```python
from build123d import *

# Parameters (mm, degrees)
BEAM_SCALE_X           = 1
BEAM_SCALE_Y           = 4
BEAM_SCALE_Z           = 1
LENGTH_SCALE_X         = 10
LENGTH_SCALE_Y         = 1
LENGTH_SCALE_Z         = 1
SKETCH6_W              = 123.825
SKETCH6_H              = 68.58
PAYLOAD_BAY_DEPTH      = 51.8000001
PAYLOAD_BAY_DEPTH_BACK = 63.5
SKETCH16_R             = 5.08
MAST_HOLE_DEPTH        = 51.8000001
MAST_HOLE_DEPTH_BACK   = 101.6
SKETCH15_2_W           = 508
SKETCH15_2_H           = 203.2
LAYER_2_DEPTH          = 50.8


with BuildPart() as part:
    # YZ Section_depthOnly → Depth (revolve)
    with BuildSketch(Plane(origin=(0, 0, 0), x_dir=(0, 0, -1), z_dir=(1, 0, 0))):
        with BuildLine():
            Line((0, 0), (0, -25.4))
            add(Edge.make_bspline(
                [(0, -25.4), (101.6, -14.816666667), (101.6, 0)],
                knots=[5.507991934, 5.507991934, 5.507991934, 6.283185307, 6.283185307, 6.283185307], degree=2, weights=[1, 0.9258201, 1]))
            Line((101.6, 0), (0, 0))
        make_face()
    revolve(axis=Axis((0, 0, 254), (0, 0, -1)))

    # Sketch13 → Height (revolve)
    with BuildSketch(Plane(origin=(0, 0, 0), x_dir=(0, 0, -1), z_dir=(1, 0, 0))):
        with BuildLine():
            Line((0, 0), (-50.8, 0))
            add(Edge.make_bspline(
                [(-50.8, 0), (-50.8, -23.988888889), (0, -25.4)],
                knots=[0, 0, 0, 1.511938821, 1.511938821, 1.511938821], degree=2, weights=[1, 0.727606875, 1]))
            Line((0, -25.4), (0, 0))
        make_face()
    revolve(axis=Axis((0, 0, 0), (0, 0, 1)))


with BuildPart() as part_1:
    # Beam: scaled about (0, 0, 0)
    add(part.part.scale((BEAM_SCALE_X, BEAM_SCALE_Y, BEAM_SCALE_Z), about=(0, 0, 0)))


with BuildPart() as part_2:
    # Length: scaled about (0, 0, 0)
    add(part_1.part.scale((LENGTH_SCALE_X, LENGTH_SCALE_Y, LENGTH_SCALE_Z), about=(0, 0, 0)))

    # Sketch6 → Payload Bay (cut, two sides)
    with BuildSketch(Plane.XY) as payload_bay_sk:
        with Locations((-74.6125, 0)):
            Rectangle(SKETCH6_W, SKETCH6_H)
        with Locations((74.6125, 0)):
            Rectangle(SKETCH6_W, SKETCH6_H)
    extrude(amount=PAYLOAD_BAY_DEPTH, mode=Mode.SUBTRACT)
    extrude(payload_bay_sk.sketch, amount=-PAYLOAD_BAY_DEPTH_BACK, mode=Mode.SUBTRACT)

    # Sketch16 → Mast Hole (cut, two sides)
    with BuildSketch(Plane.XY) as mast_hole_sk:
        Circle(SKETCH16_R)
    extrude(amount=MAST_HOLE_DEPTH, mode=Mode.SUBTRACT)
    extrude(mast_hole_sk.sketch, amount=-MAST_HOLE_DEPTH_BACK, mode=Mode.SUBTRACT)


with BuildPart() as body_2:
    # Sketch15_2 → Layer 2 (new body)
    with BuildSketch(Plane.XY):
        Rectangle(SKETCH15_2_W, SKETCH15_2_H)
    extrude(amount=-LAYER_2_DEPTH)


with BuildPart() as part_3:
    add(part_2.part)

    # Layer 2 Body: intersect body 2
    add(body_2.part, mode=Mode.INTERSECT)


solid = part_3.part
```
Build history of the part. All positions in model axes, mm. A direction names the side the tool comes from. Give positions to 0.01 mm unless a question says otherwise; leave off trailing zeros.
Item 1: Pull direction Y, two halves, no side cores. Call faces 3 (the face through (-136.525, 0, -26)), 4 (the face through (136.525, 0, -26)), 5 (the face through (-3, -16, -50.8)): released by +Y, released by -Y, zero draft, split by the parting line, or undercut.
Answers follow:
face 3: undercut
face 4: undercut
face 5: zero draft
Item 2: Slice it at A-A, the plane y = 0. Give the number of separate pieces and of enclosed holes in the cut face, and give its area (3 significant figures).
Answers follow:
separate pieces: 4
enclosed holes: 0
area: 9,580 mm2
Item 3: Flat gauge pins, fed straight in: pin 1 (2 mm diameter, centred on x = -63.5, z = -30, fed in from +Y); pin 2 (15 mm diameter, centred on y = -4, z = -34, fed in from +X); pin 3 (12 mm diameter, centred on x = 172.5, z = -19.5, fed in from -Y); pin 4 (8 mm diameter, centred on x = 0, y = 0, fed in from -Z). Where does each tip first touch, or does it go through?
Answers follow:
pin 1: stops at y = 84.17
pin 2: stops at x = 222.88
pin 3: stops at y = -66.94
pin 4: passes through
Item 4: Drill centre lines: line 1 (X direction, y = 14.5, z = -14) (3 decimals); line 2 (X direction, y = 14, z = -13) (3 decimals); line 3 (Y direction, x = 0, z = -28.5). Where is each one in solid material? Low to high.
Answers follow:
line 1: x = -235.774 to -136.525, -12.7 to 12.7, 136.525 to 235.774
line 2: x = -237.141 to -136.525, -12.7 to 12.7, 136.525 to 237.141
line 3: y = -88.17 to -5.08, 5.08 to 88.17
Item 5: Which spindle directions (+Z, -Z, +X, -X, +Y, -Y) get a long thin tool onto all of the face, cutting with end or side? Do faces 1 (the face through (-4, 5, 0)), 2 (the face through (74, 34.29, -26)). Say none if no direction does.
Answers follow:
face 1: +Z, +X, -X, +Y, -Y
face 2: +Z, -Z
